Autodesk Inventor part; units mm, degrees
ref_plane "YZ Plane" through (0, 0, 0) normal (1, 0, 0) x (0, 1, 0)
ref_plane "XZ Plane" through (0, 0, 0) normal (0, 1, 0) x (-1, 0, 0)
ref_plane "XY Plane" through (0, 0, 0) normal (0, 0, 1) x (1, 0, 0)
sketch "Sketch1" plane through (0, 0, 0) normal (0, 0, 1) x (1, 0, 0)
  line L0 (16.224, -2.484) -> (16.224, 25.338)
  line L1 (16.224, 25.338) -> (44.046, 25.338)
  line L2 (44.046, 41.562) -> (16.224, 41.562)
  line L3 (0, 41.562) -> (-27.822, 41.562)
  line L4 (-27.822, 25.338) -> (0, 25.338)
  line L5 (16.224, -2.484) -> (18.708, -2.484)
  line L6 (18.708, 44.046) -> (44.046, 44.046)
  line L7 (44.046, 22.854) -> (18.708, 22.854)
  line L8 (18.708, 22.854) -> (18.708, 0)
  line L9 (-2.484, 44.046) -> (-27.822, 44.046)
  line L10 (-27.822, 22.854) -> (-2.484, 22.854)
  line L11 (0, 0) -> (0, 25.338)
  line L12 (0, 41.562) -> (0, 71.322)
  line L13 (16.224, 71.322) -> (16.224, 41.562)
  line L14 (16.224, 25.338) -> (16.224, 0)
  line L15 (18.708, -2.484) -> (18.708, 22.854)
  line L16 (18.708, 44.046) -> (18.708, 71.322)
  line L17 (-2.484, 71.322) -> (-2.484, 44.046)
  line L18 (-2.484, 22.854) -> (-2.484, -2.484)
  line L19 (-27.822, 44.046) -> (-27.822, 41.562)
  line L20 (-27.822, 25.338) -> (-27.822, 22.854)
  line L21 (44.046, 44.046) -> (44.046, 41.562)
  line L22 (44.046, 25.338) -> (44.046, 22.854)
  line L23 (18.708, 71.322) -> (16.224, 71.322)
  line L24 (0, 71.322) -> (-2.484, 71.322)
  line L25 (-2.484, -2.484) -> (0, -2.484)
  line L26 (0, -2.484) -> (0, 1.997)
  point P0 (-25.338, 41.562)
  point P1 (-25.338, 25.338)
extrude "Extrusion1" add sketch "Sketch1" along normal blind 18
sketch "Sketch2" plane through (0, 0, 0) normal (0, 0, -1) x (-1, 0, 0)
  line L0 (2.484, 22.854) -> (2.484, -2.484)
  line L1 (27.822, 22.854) -> (2.484, 22.854)
  line L2 (27.822, 44.046) -> (27.822, 22.854)
  line L3 (2.484, 44.046) -> (27.822, 44.046)
  line L4 (2.484, 71.322) -> (2.484, 44.046)
  line L5 (-18.708, 71.322) -> (2.484, 71.322)
  line L6 (-18.708, 44.046) -> (-18.708, 71.322)
  line L7 (-44.046, 44.046) -> (-18.708, 44.046)
  line L8 (-44.046, 22.854) -> (-44.046, 44.046)
  line L9 (-18.708, 22.854) -> (-44.046, 22.854)
  line L10 (-18.708, -2.484) -> (-18.708, 22.854)
  line L11 (2.484, -2.484) -> (-18.708, -2.484)
  point P0 (0, 0)
extrude "Extrusion2" add sketch "Sketch2" along normal blind 3
sketch "Sketch3" plane through (-27.822, 44.046, 18) normal (0, 1, 0) x (1, 0, 0)
  circle A0 centre (12.6484, 10.1922) radius 1.841
  point P0 (27.822, 18)
extrude "Extrusion3" cut sketch "Sketch3" against normal blind 28
sketch "Sketch4" plane through (18.708, 44.046, 18) normal (0, 1, 0) x (1, 0, 0)
  circle A0 centre (11.4919, 10.9288) radius 1.841
  point P0 (-18.708, 18)
extrude "Extrusion4" cut sketch "Sketch4" against normal blind 28
sketch "Sketch5" plane through (18.708, 44.046, 18) normal (1, 0, 0) x (0, 0, -1)
  circle A0 centre (10.1922, -32.8499) radius 1.841
  circle A1 centre (10.1922, 13.2601) radius 1.841
  point P0 (18, -44.046)
extrude "Extrusion5" cut sketch "Sketch5" against normal blind 28
properties part number "Lifter Connecter"
Model file for the job. Use its own axes, mm. A direction names the side the tool comes from. Give positions to 0.01 mm unless a question says otherwise; leave off trailing zeros. Loops run counter-clockwise (first coordinate to the right, second up) from the corner with the lowest first, then second, coordinate; pieces in that order, holes last. Notation, with made-up numbers: (-23.75, 36) -> (-7.75, 36) arc R31 ccw to (-7.75, 68) -> close; hole circle Ø6 at (51, 62.5). An arc over 180 degrees is marked (long way). Use CSV: the item, a comma, the result in double quotes. Start each with the question number.
1) Slice it at D-D on x = 1.5. Give the cut face in (y, z).
2) Wall check: line 1 (X direction, y = 68.5, z = 2.25); line 2 (X direction, y = 43.5, z = 5.75); line 3 (Y direction, x = 24, z = 17.25). Give the ranges that are in metal, low to high.
3) Tool access for faces 5 (the flat face through (-2.484, 58, 10)), 6 (the flat face through (9, 35, 0)), 7 (the flat face through (30, 41.562, 11)), 8 (the flat face through (18.708, 10, 10)): list every direction of +Z, -Z, +X, -X, +Y, -Y with a clear straight run to the whole face (end or side of a thin tool).
4) Slice it at B-B on y = 17.5. Give the cut face in (x, z).
5) Slice it at A-A on z = 15.5. Give the cut face in (x, y), plus the area to 3 significant figures.
6) Slice it at C-C on x = 27.5. Give the cut face in (y, z).
7) Mould opens along X. For faces 1 (the flat face through (18.708, 57, 10)), 2 (the flat face through (-14, 41.562, 11)), 3 (the flat face through (16.224, 11, 11)), 4 (the cylindrical face through (-16.635, 24.113, 8.928)) say: released by +X, released by -X, zero draft, split by the parting line, or undercut.
8) Flat gauge pins, fed straight in: pin 1 Ø6 at (y, z) = (63.5, 9) entering from +X; pin 2 Ø6 at (y, z) = (57.31, 7.81) entering from -X; pin 3 Ø9 at (x, z) = (-7.5, 11) entering from +Y; pin 4 Ø4 at (x, z) = (12.5, 2.5) entering from -Y. Where does each tip first touch, or does it go through?
Computed values:
1,outline,"(-2.48, -3) -> (71.32, -3) -> (71.32, 0) -> (-2.48, 0) -> close"
2,line 1,"x = -2.48 to 0, 16.22 to 18.71"
2,line 2,"x = -27.82 to 0, 16.22 to 28.92, 31.48 to 44.05"
2,line 3,"y = 22.85 to 25.34, 41.56 to 44.05"
3,face 5,"+Z, -Z, -X, +Y"
3,face 6,"+Z"
3,face 7,"+Z, +X, -X"
3,face 8,"+Z, -Z, +X, -Y"
4,outline,"(-2.48, -3) -> (18.71, -3) -> (18.71, 18) -> (16.22, 18) -> (16.22, 0) -> (0, 0) -> (0, 18) -> (-2.48, 18) -> close"
5,outline,"(-27.82, 22.85) -> (-2.48, 22.85) -> (-2.48, -2.48) -> (0, -2.48) -> (0, 25.34) -> (-27.82, 25.34) -> close; (-27.82, 41.56) -> (0, 41.56) -> (0, 71.32) -> (-2.48, 71.32) -> (-2.48, 44.05) -> (-27.82, 44.05) -> close; (16.22, -2.48) -> (18.71, -2.48) -> (18.71, 22.85) -> (44.05, 22.85) -> (44.05, 25.34) -> (16.22, 25.34) -> close; (16.22, 41.56) -> (44.05, 41.56) -> (44.05, 44.05) -> (18.71, 44.05) -> (18.71, 71.32) -> (16.22, 71.32) -> close"
5,area,"538 mm^2"
6,outline,"(22.85, -3) -> (44.05, -3) -> (44.05, 18) -> (41.56, 18) -> (41.56, 0) -> (25.34, 0) -> (25.34, 18) -> (22.85, 18) -> close"
7,face 1,"released by +X"
7,face 2,"zero draft"
7,face 3,"undercut"
7,face 4,"undercut"
8,pin 1,"stops at x = 18.71"
8,pin 2,"stops at x = -2.48"
8,pin 3,"stops at y = 44.05"
8,pin 4,"passes through"
